```python
from build123d import *

# Parameters (mm, degrees)
SKETCH1_R             = 5.000000000000001
BOSS_EXTRUDE1_DEPTH   = 4
SKETCH1_R_2           = 5.4999999999999964
BOSS_EXTRUDE1_2_DEPTH = 4
BOSS_EXTRUDE2_DEPTH   = 2.5
SKETCH1_5_R           = 9
SKETCH1_5_R_2         = 5
BOSS_EXTRUDE3_DEPTH   = 10
SKETCH2_R             = 5.000000000000002
BOSS_EXTRUDE4_DEPTH   = 6
BOSS_EXTRUDE4_TAPER   = 10.000000000000021


with BuildPart() as part:
    # Sketch1 → Boss-Extrude1 (new, symmetric)
    with BuildSketch(Plane(origin=(0, 0, 0), x_dir=(0, 0, -1), z_dir=(1, 0, 0))):
        with Locations((-25, 0)):
            Circle(SKETCH1_R)
    extrude(amount=BOSS_EXTRUDE1_DEPTH, both=True)



with BuildPart() as body_2:
    # Sketch1 → Boss-Extrude1 2 (new, symmetric)
    with BuildSketch(Plane(origin=(0, 0, 0), x_dir=(0, 0, -1), z_dir=(1, 0, 0))):
        with Locations((40, -8)):
            Circle(SKETCH1_R_2)
    extrude(amount=BOSS_EXTRUDE1_2_DEPTH, both=True)


with BuildPart() as part_1:
    add(part.part)

    add(body_2.part)  # Boss-Extrude2 merges body 2
    # Sketch1_4 → Boss-Extrude2 (add, symmetric)
    with BuildSketch(Plane(origin=(0, 0, 0), x_dir=(0, 0, -1), z_dir=(1, 0, 0))):
        with BuildLine():
            ThreePointArc((-23.364000000000004, -4.724775550224582), (-13.97577778645901, -3.827150748913674), (-5.219999999999997, -7.331548267589863))
            ThreePointArc((-5.22, -7.331548267589868), (-8.56443458392766, 2.765946539183984), (0.05433950578730529, 8.99983595506667))
            ThreePointArc((0.05433950578730951, 8.999835955066672), (-13.442029090859073, 7.968983561268402), (-26.58726168839327, 4.741371144780544))
            ThreePointArc((-26.587261688393315, 4.7413711447806755), (-22.07906765244097, 4.058097364650495), (-20, 0))
            ThreePointArc((-20, -1.22e-15), (-20.926917629116737, -2.900000000000001), (-23.364000000000004, -4.724775550224584))
        make_face()
        with BuildLine():
            ThreePointArc((9, -2.2e-15), (7.628837505024142, -4.775022337323357), (3.933147039569554, -8.095082109844547))
            ThreePointArc((3.933147039569551, -8.095082109844547), (20.79751544110114, -5.314475765908483), (36.44338040684717, -12.195289867172626))
            ThreePointArc((36.44338040684717, -12.19528986717263), (35.55153420615901, -4.765629569602972), (42.89416462330142, -3.3230553634631823))
            ThreePointArc((42.89416462330135, -3.323055363463297), (22.323850565460532, 5.791970771239534), (0.05433950578730951, 8.999835955066672))
            ThreePointArc((0.05433950578730529, 8.99983595506667), (6.383144035351457, 6.344720027231865), (9, 0))
        make_face()
    extrude(amount=BOSS_EXTRUDE2_DEPTH, both=True)

    # Sketch1_5 → Boss-Extrude3 (add, symmetric)
    with BuildSketch(Plane(origin=(0, 0, 0), x_dir=(0, 0, -1), z_dir=(1, 0, 0))):
        Circle(SKETCH1_5_R)
        Circle(SKETCH1_5_R_2, mode=Mode.SUBTRACT)
    extrude(amount=BOSS_EXTRUDE3_DEPTH, both=True)

    # Sketch2 → Boss-Extrude4 (add)
    with BuildSketch(Plane(origin=(0, -5, 0), x_dir=(1, 0, 0), z_dir=(0, 1, 0))):
        with Locations((0, -25)):
            Circle(SKETCH2_R)
    extrude(amount=BOSS_EXTRUDE4_DEPTH, taper=BOSS_EXTRUDE4_TAPER)


solid = part_1.part
```
Could you check a few things on this model? Use its own coordinates, in mm. A direction names the side the tool comes from. Coordinates: 2 decimals unless noted, no trailing zeros. Order: outer loops, then holes, each group sorted by start corner. A loop starts at its lowest first (then second) coordinate and runs counter-clockwise, first axis right, second up. Notation, with made-up numbers: M 14.5,-13 L 50.5,-13 A17 ccw 50.5,12 Z; hole C 83,-0.5 d2. An arc over 180 degrees is marked long. Use a Markdown table: item, result. Add a question column.
Q1. I want a section at B-B on x = 0. List the corners of the cut face in (y, z) for me, then the cut area to 3 significant figures.
Q2. Which directions (+Z, -Z, +X, -X, +Y, -Y) give clear straight access to the entire face, cutting with the end or side of a thin tool? Please do faces 1 (the cylindrical face through (0.06, -10.11, -45.08)), 2 (the flat face through (-4, 1, 25)), 3 (the flat face through (0, -5, 25)), 4 (the flat face through (-4, -8, -40)), 5 (the flat face through (4, -8, -40)).
Q3. If I drill on L1, parallel to Y at x = 4.5, z = 0; L2, parallel to X at y = -7.75, z = -36.5; L3, parallel to X at y = 3.5, z = -24.5, over which ranges is the centre line in solid material (lowest first)?
Q4. I want a section at C-C on z = 6. List the corners of the cut face in (x, y) for me, then the cut area to 3 significant figures.
Q5. I want a section at A-A on y = 0. List the corners of the cut face in (x, z) for me, then the cut area to 3 significant figures.
Q6. I want a section at D-D on x = -6.25. List the corners of the cut face in (y, z) for me.
Q7. I'm going to push flat-ended pins straight in: pin 1 (9 mm diameter, centred on y = -9.5, z = -42, fed in from +X); pin 2 (1 mm diameter, centred on x = -6, y = -8, fed in from -Z); pin 3 (8 mm diameter, centred on x = -1, z = 27, fed in from -Y); pin 4 (13 mm diameter, centred on y = 0, z = 0, fed in from -X). Where does each tip first touch, or does it pass through?
Checked values:
| question | item | result |
|---|---|---|
| 1 | outline | M -12.2,-36.44 A5.5 ccw long -3.32,-42.89 A82.36 ccw 4.74,26.59 A5 ccw -2.18,29.5 L -5,30 L -5,20 L -3.91,20.19 A20 cw -7.33,5.22 A9 ccw -8.1,-3.93 A30 cw Z; hole C 0,0 d10 |
| 1 | area | 868 mm² |
| 2 | face 1 | none |
| 2 | face 2 | -X, +Y |
| 2 | face 3 | +Z, +X, -X, -Y |
| 2 | face 4 | -Z, -X, +Y, -Y |
| 2 | face 5 | -Z, +X, +Y, -Y |
| 3 | L1 | -9 to -5, 5 to 9 |
| 3 | L2 | -4 to 4 |
| 3 | L3 | -2.5 to 2.5 |
| 4 | outline | M -10,-6.71 L -2.5,-6.71 L -2.5,-6.8 L 2.5,-6.8 L 2.5,-6.71 L 10,-6.71 L 10,6.71 L 2.5,6.71 L 2.5,8.81 L -2.5,8.81 L -2.5,6.71 L -10,6.71 Z |
| 4 | area | 279 mm² |
| 5 | outline | M -10,-9 L -2.5,-9 L -2.5,-37 L 2.5,-37 L 2.5,-9 L 10,-9 L 10,-5 L -10,-5 Z; M -10,5 L 10,5 L 10,9 L 2.5,9 L 2.5,20 L 4,20 L 4,24.02 A4.12 ccw 4,25.98 L 4,30 L -4,30 L -4,25.98 A4.12 ccw -4,24.02 L -4,20 L -2.5,20 L -2.5,9 L -10,9 Z |
| 5 | area | 435 mm² |
| 6 | outline | C 0,0 d18; hole C 0,0 d10 |
| 7 | pin 1 | x = 4 |
| 7 | pin 2 | z = -4.97 |
| 7 | pin 3 | y = -5 |
| 7 | pin 4 | x = -10 |
